```python
from build123d import *

# Parameters (mm, degrees)
F0_W     = 63.5
F0_H     = 82.55
F0_R     = 2.5
F0_R_2   = 12.7
F1_DEPTH = 4.7625
F2_DEPTH = 152.4
F3_DEPTH = 50.8
F4_DEPTH = 7.05
F5_DEPTH = 7.05
F6_R     = 3
F7_SIZE2 = 20
F7_SIZE  = 45
F8_SIZE2 = 20
F8_SIZE  = 45


with BuildPart() as f1:
    # F0 (on Top) → F1 (new body)
    with BuildSketch(Plane.XY):
        Rectangle(F0_W, F0_H)
        with Locations((-20.6375, -31.75)):
            Circle(F0_R, mode=Mode.SUBTRACT)
        with Locations((20.6375, -31.75)):
            Circle(F0_R, mode=Mode.SUBTRACT)
        with Locations((-20.6375, 25.4)):
            Circle(F0_R, mode=Mode.SUBTRACT)
        with Locations((-20.6375, 31.75)):
            Circle(F0_R, mode=Mode.SUBTRACT)
        with BuildLine():
            ThreePointArc((1.5875, 14.1990316571), (10.6492737428, 9.525), (14.2875, 0))
            ThreePointArc((14.2875, 0), (10.6492737428, -9.525), (1.5875, -14.1990316571))
            Line((1.5875, -14.1990316571), (1.5875, -31.75))
            Line((1.5875, -31.75), (0, -31.75))
            Line((0, -31.75), (-1.5875, -31.75))
            Line((-1.5875, -31.75), (-1.5875, -14.1990316571))
            ThreePointArc((-1.5875, -14.1990316571), (-14.2875, 0), (-1.5875, 14.1990316571))
            Line((-1.5875, 14.1990316571), (-1.5875, 31.75))
            Line((-1.5875, 31.75), (0, 31.75))
            Line((0, 31.75), (1.5875, 31.75))
            Line((1.5875, 31.75), (1.5875, 14.1990316571))
        make_face(mode=Mode.SUBTRACT)
        with Locations((20.6375, 25.4)):
            Circle(F0_R, mode=Mode.SUBTRACT)
        with Locations((20.6375, 31.75)):
            Circle(F0_R, mode=Mode.SUBTRACT)
        with BuildLine():
            Line((1.5875, -31.75), (1.5875, -14.1990316571))
            ThreePointArc((1.5875, -14.1990316571), (0, -14.2875), (-1.5875, -14.1990316571))
            Line((-1.5875, -14.1990316571), (-1.5875, -31.75))
            Line((-1.5875, -31.75), (0, -31.75))
            Line((0, -31.75), (1.5875, -31.75))
        make_face()
        with BuildLine():
            ThreePointArc((1.5875, -14.1990316571), (10.6492737428, -9.525), (14.2875, 0))
            ThreePointArc((14.2875, 0), (10.6492737428, 9.525), (1.5875, 14.1990316571))
            ThreePointArc((1.5875, 14.1990316571), (0, 14.2875), (-1.5875, 14.1990316571))
            ThreePointArc((-1.5875, 14.1990316571), (-14.2875, 0), (-1.5875, -14.1990316571))
            ThreePointArc((-1.5875, -14.1990316571), (0, -14.2875), (1.5875, -14.1990316571))
        make_face()
        Circle(F0_R_2, mode=Mode.SUBTRACT)
        Circle(F0_R_2)
        Circle(F0_R, mode=Mode.SUBTRACT)
        with BuildLine():
            ThreePointArc((-1.5875, 14.1990316571), (0, 14.2875), (1.5875, 14.1990316571))
            Line((1.5875, 14.1990316571), (1.5875, 31.75))
            Line((1.5875, 31.75), (0, 31.75))
            Line((0, 31.75), (-1.5875, 31.75))
            Line((-1.5875, 31.75), (-1.5875, 14.1990316571))
        make_face()
        with Locations((-20.6375, 25.4)):
            Circle(F0_R)
        with Locations((20.6375, 25.4)):
            Circle(F0_R)
    extrude(amount=-F1_DEPTH)

    # F0 (on Top) → F2 (join)
    with BuildSketch(Plane.XY):
        with BuildLine():
            ThreePointArc((1.5875, -14.1990316571), (10.6492737428, -9.525), (14.2875, 0))
            ThreePointArc((14.2875, 0), (10.6492737428, 9.525), (1.5875, 14.1990316571))
            ThreePointArc((1.5875, 14.1990316571), (0, 14.2875), (-1.5875, 14.1990316571))
            ThreePointArc((-1.5875, 14.1990316571), (-14.2875, 0), (-1.5875, -14.1990316571))
            ThreePointArc((-1.5875, -14.1990316571), (0, -14.2875), (1.5875, -14.1990316571))
        make_face()
        Circle(F0_R_2, mode=Mode.SUBTRACT)
    extrude(amount=F2_DEPTH)

    # F0 (on Top) → F3 (join)
    with BuildSketch(Plane.XY):
        with BuildLine():
            Line((1.5875, -31.75), (1.5875, -14.1990316571))
            ThreePointArc((1.5875, -14.1990316571), (0, -14.2875), (-1.5875, -14.1990316571))
            Line((-1.5875, -14.1990316571), (-1.5875, -31.75))
            Line((-1.5875, -31.75), (0, -31.75))
            Line((0, -31.75), (1.5875, -31.75))
        make_face()
        with BuildLine():
            ThreePointArc((-1.5875, 14.1990316571), (0, 14.2875), (1.5875, 14.1990316571))
            Line((1.5875, 14.1990316571), (1.5875, 31.75))
            Line((1.5875, 31.75), (0, 31.75))
            Line((0, 31.75), (-1.5875, 31.75))
            Line((-1.5875, 31.75), (-1.5875, 14.1990316571))
        make_face()
    extrude(amount=F3_DEPTH)

    # F4 (add): a face of the model
    f4_faces = [f1.faces().sort_by_distance(p)[0] for p in [
        (0, -31.75, 25.4),
    ]]
    extrude(f4_faces, amount=F4_DEPTH)

    # F5 (add): a face of the model
    f5_faces = [f1.faces().sort_by_distance(p)[0] for p in [
        (0, 31.75, 25.4),
    ]]
    extrude(f5_faces, amount=F5_DEPTH)

    # F6
    f6_edges = [f1.edges().sort_by_distance(p)[0] for p in [
        (31.75, -41.275, -2.38125),
        (31.75, 41.275, -2.38125),
        (-31.75, 41.275, -2.38125),
        (-31.75, -41.275, -2.38125),
    ]]
    fillet(f6_edges, radius=F6_R)

    # F7
    f7_edges = [f1.edges().sort_by_distance(p)[0] for p in [
        (0, -38.8, 50.8),
    ]]
    f7_side = f1.faces().sort_by_distance((0, -38.8, 25.4))[0]
    chamfer(f7_edges, length=F7_SIZE, length2=F7_SIZE2, reference=f7_side)

    # F8
    f8_edges = [f1.edges().sort_by_distance(p)[0] for p in [
        (0, 38.8, 50.8),
    ]]
    chamfer(f8_edges, length=F8_SIZE, length2=F8_SIZE2)


solid = f1.part
```
Could you check a few things on this model? Use its own coordinates, in mm. A direction names the side the tool comes from. Coordinates: 2 decimals unless noted, no trailing zeros. Write each loop counter-clockwise with the first axis right and the second up, starting at its lowest first coordinate (ties: lowest second). Pieces come first, ordered by that corner, then holes. Notation, with made-up numbers: (71, 31.25) -> (107, 31.25) arc R30 cw to (107, 61.25) -> close; hole circle Ø2 at (83, 12.25). An arc over 180 degrees is marked (long way). Write item = value, one per line. Start each with the question number.
(1) I need wall thicknesses on line 1 (Y direction, x = 0, z = 119.5); line 2 (X direction, y = 31, z = -2); line 3 (Z direction, x = -27.5, y = 32). Which ranges of each line are inside material? Lowest first, please. Write a range as [from, to].
(2) I want a section at D-D (y = -31.75). Please give me the cut outline in (x, z), plus the area to 3 significant figures.
(3) I want a section at B-B (y = 36). Please give me the cut outline in (x, z), plus the area to 3 significant figures.
(4) We'd pull the mould along Y, two halves only. Please class faces 1 (the face through (0, 41.275, -2)), 2 (the face through (20.31, -29.27, -2.35)), 3 (the face through (0, -41.275, -2)): released by +Y, released by -Y, zero draft, split by the parting line, or undercut.
(5) Which directions (+Z, -Z, +X, -X, +Y, -Y) give clear straight access to the entire face, cutting with the end or side of a thin tool? Please do faces 4 (the face through (-1.588, 24, 19)), 5 (the face through (-1.588, -24, 19)), 6 (the face through (1.588, -24, 19)), 7 (the face through (1.588, 24, 19)).
(6) Will these pins go through, and if not, where does the flat tip stop? pin 1 (7.5 mm diameter, centred on y = -30, z = 28.5, fed in from +X); pin 2 (3 mm diameter, centred on y = -5, z = 96.5, fed in from +X); pin 3 (12 mm diameter, centred on x = -22.5, y = -1.5, fed in from +Z).
(7) I want a section at A-A (x = 0). Please give me the cut outline in (y, z) (1 decimal).
(8) I want a section at C-C (z = 141.5). Please give me the cut outline in (x, y) (1 decimal).
Result set:
q1.line_1 = [-14.29, -12.7], [12.7, 14.29]
q1.line_2 = [-31.75, -23.02], [-18.25, 18.25], [23.02, 31.75]
q1.line_3 = [-4.76, 0]
q2.outline = (-31.75, -4.76) -> (-23.14, -4.76) -> (-23.14, 0) -> (-31.75, 0) -> close; (-18.14, -4.76) -> (18.14, -4.76) -> (18.14, 0) -> (1.59, 0) -> (1.59, 21.66) -> (-1.59, 21.66) -> (-1.59, 0) -> (-18.14, 0) -> close; (23.14, -4.76) -> (31.75, -4.76) -> (31.75, 0) -> (23.14, 0) -> close
q2.area = 324 mm2
q3.outline = (-31.75, -4.76) -> (31.75, -4.76) -> (31.75, 0) -> (1.59, 0) -> (1.59, 12.1) -> (-1.59, 12.1) -> (-1.59, 0) -> (-31.75, 0) -> close
q3.area = 341 mm2
q4.face_1 = released by +Y
q4.face_2 = undercut
q4.face_3 = released by -Y
q5.face_4 = +Z, -X, +Y
q5.face_5 = +Z, -X, -Y
q5.face_6 = +Z, +X, -Y
q5.face_7 = +Z, +X, +Y
q6.pin_1 = 1.59
q6.pin_2 = 13.85
q6.pin_3 = 0
q7.outline = (-41.3, -4.8) -> (-2.5, -4.8) -> (-2.5, 0) -> (-12.7, 0) -> (-12.7, 152.4) -> (-14.3, 152.4) -> (-14.3, 50.8) -> (-18.8, 50.8) -> (-38.8, 5.8) -> (-38.8, 0) -> (-41.3, 0) -> close; (2.5, -4.8) -> (41.3, -4.8) -> (41.3, 0) -> (38.8, 0) -> (38.8, 5.8) -> (18.8, 50.8) -> (14.3, 50.8) -> (14.3, 152.4) -> (12.7, 152.4) -> (12.7, 0) -> (2.5, 0) -> close
q8.outline = circle Ø28.6 at (0, 0); hole circle Ø25.4 at (0, 0)
